Source: CAD feature listing. Evaluate the final solid. Frame: model axes, mm. A direction names the side the tool comes from. Give positions to 0.01 mm unless a question says otherwise; leave off trailing zeros. Loops run counter-clockwise (first coordinate to the right, second up) from the corner with the lowest first, then second, coordinate; pieces in that order, holes last. Notation, with made-up numbers: (21.5, 27) -> (63.5, 27) arc R15 cw to (63.5, 45) -> close; hole circle Ø11 at (54, 80). An arc over 180 degrees is marked (long way). Return JSON: item names as keys, results as strings. Group by question number.
```python
from build123d import *

# Parameters (mm, degrees)
SKETCH1_R           = 12.5
BOSS_EXTRUDE1_DEPTH = 150
SKETCH2_W           = 8.15
SKETCH2_H           = 8.15
BOSS_EXTRUDE2_DEPTH = 12
FILLET1_R           = 3
SKETCH3_W           = 8.2
SKETCH3_H           = 8.2
CUT_EXTRUDE1_DEPTH  = 20


with BuildPart() as part:
    # Sketch1 → Boss-Extrude1 (new body)
    with BuildSketch(Plane(origin=(0, 0, 0), x_dir=(1, 0, 0), z_dir=(0, 1, 0))):
        Circle(SKETCH1_R)
    extrude(amount=BOSS_EXTRUDE1_DEPTH)

    # Sketch2 → Boss-Extrude2 (add)
    with BuildSketch(Plane(origin=(0, 150, 0), x_dir=(1, 0, 0), z_dir=(0, 1, 0))):
        Rectangle(SKETCH2_W, SKETCH2_H)
    extrude(amount=BOSS_EXTRUDE2_DEPTH)

    # Fillet1
    fillet1_edges = [part.edges().sort_by_distance(p)[0] for p in [
        (4.075, 162, 0),
        (0, 162, -4.075),
        (-4.075, 162, 0),
        (0, 162, 4.075),
    ]]
    fillet(fillet1_edges, radius=FILLET1_R)

    # Sketch3 → Cut-Extrude1 (cut)
    with BuildSketch(Plane.XZ):
        Rectangle(SKETCH3_W, SKETCH3_H)
    extrude(amount=-CUT_EXTRUDE1_DEPTH, mode=Mode.SUBTRACT)


solid = part.part
```
1) Material intervals for line 1 (X direction, y = 12, z = -0.5); line 2 (Y direction, x = 9, z = 2.75); line 3 (Z direction, x = 6.75, y = 70.5), sorted ascending.
2) Cut plane A-A on y = 99. Return loops of the section in (x, z), then the cut area to 3 significant figures.
3) Cut plane B-B on z = 8. Return loops of the section in (x, y), then the cut area to 3 significant figures.
4) Reachability of faces 5 (the face through (-4.1, 10, 0)), 6 (the face through (0, 154, -4.075)), 7 (the face through (-4.075, 154, 0)) from +Z, -Z, +X, -X, +Y, -Y: full face, straight path, thin tool, end or side. Return the list, or none.
5) Contact query for flat-ended pins moving along their axis: P1, Ø9, axis at x = -2, y = 155, coming from the -Z side (3 decimals); P2, Ø5, axis at y = 46.5, z = 9.5, coming from the +X side; P3, Ø3, axis at x = -1, z = 2, coming from the -Y side. Output: stop coordinate, or through.
6) Mould query, pull axis Z, two halves, no side actions, for faces 1 (the face through (0.057, 160.694, -3.551)), 2 (the face through (-3.551, 160.694, -0.057)), 3 (the face through (0, 154, 4.075)), 4 (the face through (0, 10, -4.1)). Classes: released by +Z, released by -Z, zero draft, split by the parting line, or undercut.
Calculated:
{
 "1": {"line 1": "-12.49 to -4.1, 4.1 to 12.49", "line 2": "0 to 150", "line 3": "-10.52 to 10.52"},
 "2": {"outline": "circle Ø25 at (0, 0)", "area": "491 mm2"},
 "3": {"outline": "(-9.6, 0) -> (9.6, 0) -> (9.6, 150) -> (-9.6, 150) -> close", "area": "2,880 mm2"},
 "4": {"face 5": "-Y", "face 6": "-Z, +X, -X, +Y", "face 7": "+Z, -Z, -X, +Y"},
 "5": {"P1": "z = -4.075", "P2": "x = 10.36", "P3": "y = 20"},
 "6": {"face 1": "released by -Z", "face 2": "zero draft", "face 3": "released by +Z", "face 4": "undercut"}
}
